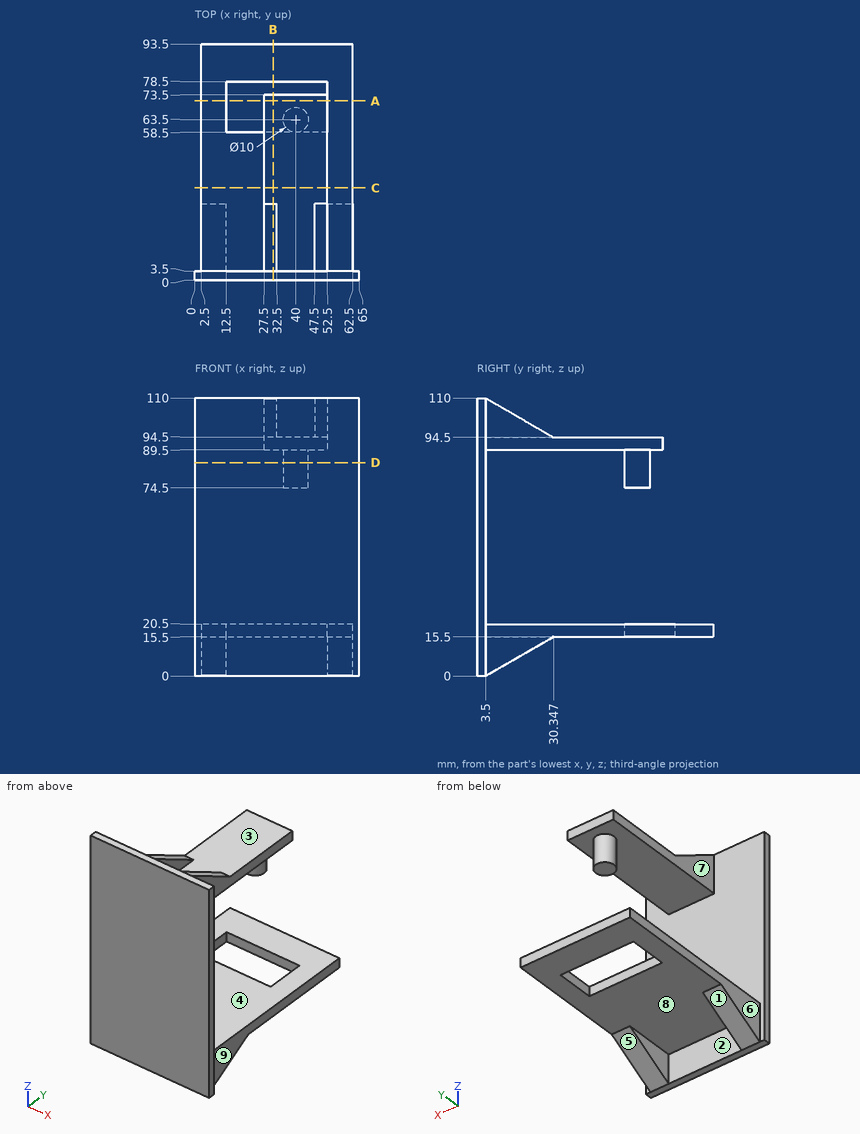
Geometry check sheet. Reference: drawing and pictorial views, mm from the part's lowest x, y, z. A direction names the side the tool comes from. Give positions to 0.01 mm unless a question says otherwise; leave off trailing zeros. Order: outer loops, then holes, each group sorted by start corner. A loop starts at its lowest first (then second) coordinate and runs counter-clockwise, first axis right, second up. Notation, with made-up numbers: M -21,70.5 L -8,70.5 A29 cw -8,96.5 Z; hole C -13.75,59.25 d7. An arc over 180 degrees is marked long. Return JSON: item names as keys, results as strings. Group by question number.
1) Section check B-B on x = 31. Record the cut outline in (y, z).
2) Access from +Z, -Z, +X, -X, +Y, -Y to the whole of each face (thin tool, end or side, straight path). Record for the marked faces 5, 6, 7, 8 and 9.
3) Section check C-C on y = 36.5. Record the cut outline in (x, z).
4) Mould release check, pull along Z, two halves, no side actions. Record for the marked faces 1, 2, 3 and 4: pulls with the +Z half, pulls with the -Z half, needs draft (parallel to the pull), parting line crosses it, or undercut.
5) Go/stop test with flat-tipped pins: pin 1 Ø7.5 at (x, y) = (42.5, 39.5) entering from -Z; pin 2 Ø17 at (y, z) = (21, 11) entering from +X; pin 3 Ø3 at (x, z) = (13, 87.5) entering from +Y. Record where each tip stops, or that it passes through.
6) Section check D-D on z = 84.5. Record the cut outline in (x, y), and give its area (3 significant figures).
7) Scan lines: line 1 (X direction, y = 13.5, z = 95); line 2 (Z direction, x = 29, y = 41.5); line 3 (Z direction, x = 19, y = 9.5). Record each from-to range of solid material in increasing order.
8) Section check A-A on y = 71. Record the cut outline in (x, z).
Answer block:
{
 "1": {"outline": "M 0,0 L 3.5,0 L 3.5,15.5 L 58.5,15.5 L 58.5,20.5 L 3.5,20.5 L 3.5,89.5 L 73.5,89.5 L 73.5,94.5 L 30.35,94.5 L 3.5,110 L 0,110 Z; M 78.5,15.5 L 93.5,15.5 L 93.5,20.5 L 78.5,20.5 Z"},
 "2": {"face 5": "-Z, +X, -X, +Y", "face 6": "+Z, -Z, -X, +Y", "face 7": "+Z, -X, +Y", "face 8": "-Z, +Y", "face 9": "+Z, -Z, +X, +Y"},
 "3": {"outline": "M 2.5,15.5 L 62.5,15.5 L 62.5,20.5 L 2.5,20.5 Z; M 27.5,89.5 L 52.5,89.5 L 52.5,94.5 L 27.5,94.5 Z"},
 "4": {"face 1": "pulls with the -Z half", "face 2": "needs draft", "face 3": "pulls with the +Z half", "face 4": "undercut"},
 "5": {"pin 1": "stops at z = 15.5", "pin 2": "stops at x = 62.5", "pin 3": "stops at y = 3.5"},
 "6": {"outline": "M 0,0 L 65,0 L 65,3.5 L 0,3.5 Z; C 40,63.5 d10", "area": "306 mm^2"},
 "7": {"line 1": "x = 27.5 to 32.5, 47.5 to 52.5", "line 2": "z = 15.5 to 20.5, 89.5 to 94.5", "line 3": "z = 15.5 to 20.5"},
 "8": {"outline": "M 2.5,15.5 L 12.5,15.5 L 12.5,20.5 L 2.5,20.5 Z; M 27.5,89.5 L 52.5,89.5 L 52.5,94.5 L 27.5,94.5 Z; M 52.5,15.5 L 62.5,15.5 L 62.5,20.5 L 52.5,20.5 Z"}
}
